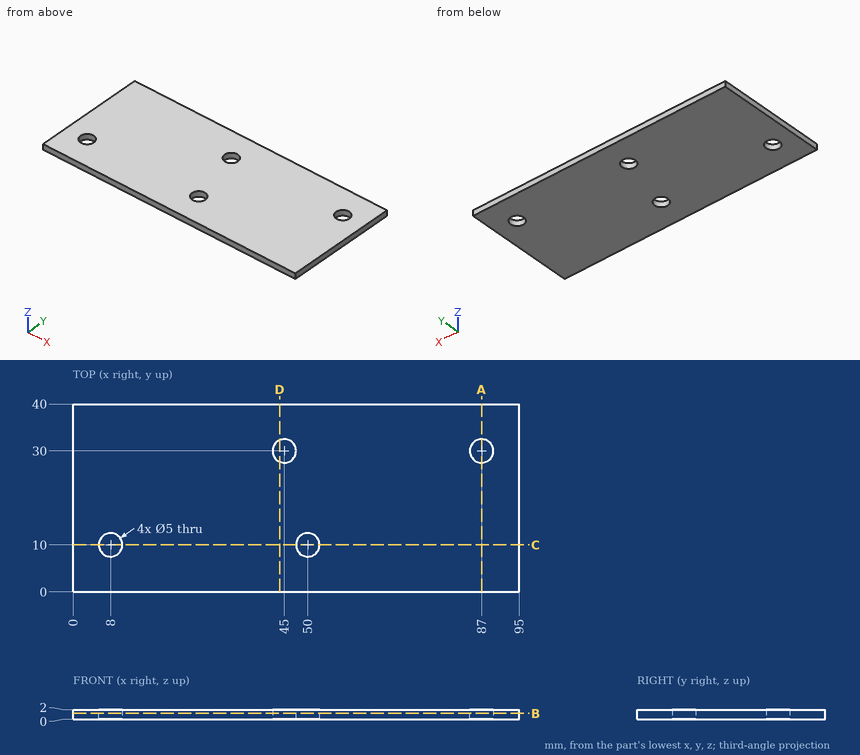
Geometry: see drawing. Coordinates: mm, zero at the bounding-box minimum. Round coordinates to 2 decimals unless told otherwise and drop trailing zeros. Loops run counter-clockwise (first coordinate to the right, second up) from the corner with the lowest first, then second, coordinate; pieces in that order, holes last. Notation, with made-up numbers: M 44,51.25 L 94,51.25 A15 ccw 94,73.25 Z; hole C 38.25,0 d9. An arc over 180 degrees is marked long. Use a Markdown table: item, result. Add a question column.
1. Line query: line 1 (Y direction, x = 8, z = 1.2); line 2 (Y direction, x = 87, z = 1.05). Output: solid intervals per line, ascending.
2. Section query A-A on x = 87. Return the cut outline in (y, z).
3. Section query B-B on z = 1.25. Return the cut outline in (x, y).
4. Section query D-D on x = 44. Return the cut outline in (y, z), then the cut area to 3 significant figures.
5. Contact query for a flat-ended pin moving along its axis: P1, Ø4.5, axis at x = 8, y = 10, coming from the -Z side. Output: stop coordinate, or through.
6. Section query C-C on y = 10. Return the cut outline in (x, z), then the cut area to 3 significant figures.
Reported:
| question | item | result |
|---|---|---|
| 1 | line 1 | y = 0 to 7.5, 12.5 to 40 |
| 1 | line 2 | y = 0 to 27.5, 32.5 to 40 |
| 2 | outline | M 0,0 L 27.5,0 L 27.5,2 L 0,2 Z; M 32.5,0 L 40,0 L 40,2 L 32.5,2 Z |
| 3 | outline | M 0,0 L 95,0 L 95,40 L 0,40 Z; hole C 8,10 d5; hole C 45,30 d5; hole C 50,10 d5; hole C 87,30 d5 |
| 4 | outline | M 0,0 L 27.71,0 L 27.71,2 L 0,2 Z; M 32.29,0 L 40,0 L 40,2 L 32.29,2 Z |
| 4 | area | 70.8 mm² |
| 5 | P1 | passes through |
| 6 | outline | M 0,0 L 5.5,0 L 5.5,2 L 0,2 Z; M 10.5,0 L 47.5,0 L 47.5,2 L 10.5,2 Z; M 52.5,0 L 95,0 L 95,2 L 52.5,2 Z |
| 6 | area | 170 mm² |
